```python
from build123d import *

# Parameters (mm, degrees)
F1_DEPTH = 2
F3_DEPTH = 2
F4_R     = 1


with BuildPart() as f1:
    # F0 (on Top) → F1 (new body)
    with BuildSketch(Plane.XY):
        Polygon((0, 3), (0, 0), (12, 0), (12, 3), (0, 6), align=None)
    extrude(amount=F1_DEPTH)

    # F2 (on face) → F3 (join, through all)
    with BuildSketch(Plane.XY.offset(2)):
        Polygon((15, 3), (12, 3), (12, 0), (12, -6), (15, -6), align=None)
    extrude(amount=-F3_DEPTH)

    # F4
    f4_edges = [f1.edges().sort_by_distance(p)[0] for p in [
        (12, 0, 1),
        (12, 3, 1),
        (15, 3, 1),
    ]]
    fillet(f4_edges, radius=F4_R)


solid = f1.part
```
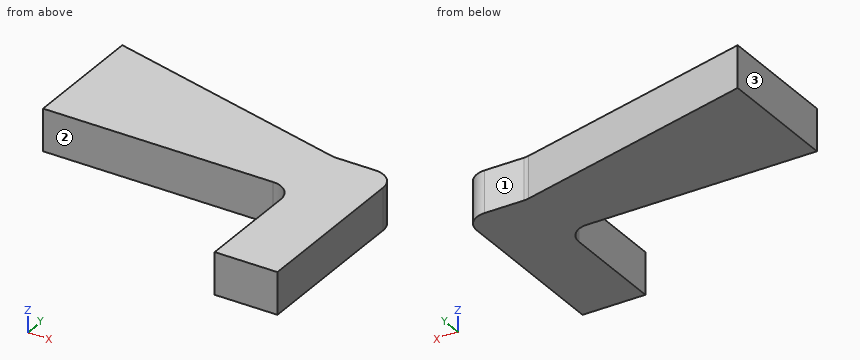
Could you check a few things on this model? Use its own coordinates, in mm. Face numbers are marked on the shaded views. A direction names the side the tool comes from. Give positions to 0.01 mm unless a question says otherwise; leave off trailing zeros. Loops run counter-clockwise (first coordinate to the right, second up) from the corner with the lowest first, then second, coordinate; pieces in that order, holes last. Notation, with made-up numbers: (67, 22) - (122, 22) arc R35 cw to (122, 56) - close; hole circle Ø6 at (63, -39.75). An arc over 180 degrees is marked (long way). Use one line per item in the form item = value.
1. I want a section at C-C (y = -3.75). Please give me the cut outline in (x, z), and give its area (3 significant figures).
Response values:
outline = (12, 0) - (15, 0) - (15, 2) - (12, 2) - close
area = 6.00 mm²
2. I need wall thicknesses on probe 1 along Y at (x, z) = (13, 1.7); probe 2 along X at (y, z) = (-4.5, 1.75); probe 3 along Y at (x, z) = (10.5, 1.2) (3 decimals). Which ranges of each line are inside material? Lowest first, please.
Response values:
probe_1 = -6 to 3
probe_2 = 12 to 15
probe_3 = 0 to 3.375
3. I'm going to push flat-ended pins straight in: pin 1 Ø0.9 at (x, z) = (13, 1.5) entering from +Y; pin 2 Ø1 at (x, z) = (7.5, 1) entering from -Y. Where does each tip first touch, or does it pass through?
Response values:
pin_1 = 3
pin_2 = 0
4. I want a section at B-B (x = 9). Please give me the cut outline in (y, z).
Response values:
outline = (0, 0) - (3.75, 0) - (3.75, 2) - (0, 2) - close
5. I want a section at A-A (z = 0.4). Please give me the cut outline in (x, y), and give its area (3 significant figures).
Response values:
outline = (0, 0) - (11, 0) arc R1 cw to (12, -1) - (12, -6) - (15, -6) - (15, 2) arc R1 ccw to (14, 3) - (12.12, 3) arc R1 cw to (11.88, 3.03) - (0, 6) - close
area = 81.0 mm²
6. On a 3-axis mill with a long thin cutter (end or side, diameter ignored), from which of +Z, -Z, +X, -X, +Y, -Y can I reach the whole of each face in a straight line? I mean the marked faces 1, 2 and 3. Say none if no direction works.
Response values:
face_1 = +Z, -Z, +X, +Y
face_2 = +Z, -Z, -X, -Y
face_3 = +Z, -Z, -X, +Y, -Y
